```python
from build123d import *

# Parameters (mm, degrees)
ESBO_O1_R                = 175
RESSALTO_EXTRUS_O1_DEPTH = 97.5
ESBO_O4_R                = 1.5
ESBO_O4_R_2              = 2
CORTE_EXTRUS_O1_DEPTH    = 10
ESBO_O5_OUTSIDE_W        = 452.898
ESBO_O5_OUTSIDE_H        = 452.898
CORTE_EXTRUS_O2_DEPTH    = 8.4


with BuildPart() as part:
    # Esboço1 → Ressalto-extrusão1 (new body)
    with BuildSketch(Plane.XY):
        Circle(ESBO_O1_R)
    extrude(amount=RESSALTO_EXTRUS_O1_DEPTH)

    # Esboço4 → Corte-extrusão1 (cut)
    with BuildSketch(Plane.XY.offset(97.5)):
        with Locations((-120, 82)):
            Circle(ESBO_O4_R)
        with Locations((-55, 120)):
            Circle(ESBO_O4_R)
        with Locations((-77, 111.8)):
            Circle(ESBO_O4_R)
        with Locations((55, 120)):
            Circle(ESBO_O4_R)
        with Locations((-7, 111.8)):
            Circle(ESBO_O4_R_2)
        with Locations((-73, 80)):
            Circle(ESBO_O4_R_2)
        with Locations((21, 80)):
            Circle(ESBO_O4_R_2)
        with Locations(Location((21, -80, 0), (0, 0, 180))):
            Circle(ESBO_O4_R_2)
        with Locations(Location((-73, -80, 0), (0, 0, 180))):
            Circle(ESBO_O4_R_2)
        with Locations(Location((-7, -111.8, 0), (0, 0, 180))):
            Circle(ESBO_O4_R_2)
        with Locations(Location((55, -120, 0), (0, 0, 180))):
            Circle(ESBO_O4_R)
        with Locations(Location((-77, -111.8, 0), (0, 0, 180))):
            Circle(ESBO_O4_R)
        with Locations(Location((-55, -120, 0), (0, 0, 180))):
            Circle(ESBO_O4_R)
        with Locations(Location((-120, -82, 0), (0, 0, 180))):
            Circle(ESBO_O4_R)
    extrude(amount=-CORTE_EXTRUS_O1_DEPTH, mode=Mode.SUBTRACT)

    # Esboço5 outside → Corte-extrusão2 (cut)
    with BuildSketch(Plane.XY.offset(97.5)):
        Rectangle(ESBO_O5_OUTSIDE_W, ESBO_O5_OUTSIDE_H)
        with BuildLine():
            Line((28, -155.307222412), (120.5, -101.902322512))
            ThreePointArc((120.5, -101.902322512), (140.997422612, -81.4048999), (148.5, -53.4048999))
            Line((148.5, -53.4048999), (148.5, 53.4048999))
            ThreePointArc((148.5, 53.4048999), (140.997422612, 81.4048999), (120.5, 101.902322512))
            Line((120.5, 101.902322512), (28, 155.307222412))
            ThreePointArc((28, 155.307222412), (0, 162.8097998), (-28, 155.307222412))
            Line((-28, 155.307222412), (-120.5, 101.902322512))
            ThreePointArc((-120.5, 101.902322512), (-140.997422612, 81.4048999), (-148.5, 53.4048999))
            Line((-148.5, 53.4048999), (-148.5, -53.4048999))
            ThreePointArc((-148.5, -53.4048999), (-140.997422612, -81.4048999), (-120.5, -101.902322512))
            Line((-120.5, -101.902322512), (-28, -155.307222412))
            ThreePointArc((-28, -155.307222412), (0, -162.8097998), (28, -155.307222412))
        make_face(mode=Mode.SUBTRACT)
    extrude(amount=-CORTE_EXTRUS_O2_DEPTH, mode=Mode.SUBTRACT)


solid = part.part
```
Design review of the part built by this model. Coordinates are the model's own, in mm. A direction names the side the tool comes from. Give positions to 0.01 mm unless a question says otherwise; leave off trailing zeros. Write each loop counter-clockwise with the first axis right and the second up, starting at its lowest first coordinate (ties: lowest second). Pieces come first, ordered by that corner, then holes. Notation, with made-up numbers: (-1, 43.5) - (13, 43.5) arc R27 ccw to (13, 82.5) - close; hole circle Ø10 at (-17, -10). An arc over 180 degrees is marked (long way). Return JSON: item names as keys, results as strings. Group by question number.
(1) We need section C-C, the plane x = 139.5. Give the boundary of the cut face in (y, z).
(2) We need section B-B, the plane z = 39. Give the boundary of the cut face in (x, y), then the cut area to 3 significant figures.
(3) Machinability: for faces 1 (the flat face through (148.5, -1, 93)), 2 (the flat face through (73.6, -128.98, 93.36)), 3 (the flat face through (-79, -129, 89.1)), 4 (the cylindrical face through (-141.2, -81.05, 93.36)), which of the approach directions +Z, -Z, +X, -X, +Y, -Y give a long, thin tool a straight path to every point of the face, cutting with its end or side? Answer none if there is none.
(4) To check wall thickness, follow probe 1 along Y at (x, z) = (21, 93.25); probe 2 along X at (y, z) = (111, 90); probe 3 along Y at (x, z) = (-120, 93). State the ranges of each line that lie inside material, in increasing order.
(5) Insertion check: pin 1 (1.5 mm diameter, centred on x = 55.5, y = 120, fed in from +Z); pin 2 (4 mm diameter, centred on x = -9, z = 10, fed in from +Y); pin 3 (5 mm diameter, centred on x = -115.5, z = 49, fed in from -Y). Each pin has a flat end and moves straight along its axis. Give the tip position at first contact, or say it passes through.
(6) We need section A-A, the plane y = 39. Give the boundary of the cut face in (x, z).
Reported:
{
 "1": {"outline": "(-105.66, 0) - (105.66, 0) - (105.66, 89.1) - (83.85, 89.1) - (83.85, 97.5) - (-83.85, 97.5) - (-83.85, 89.1) - (-105.66, 89.1) - close"},
 "2": {"outline": "circle Ø350 at (0, 0)", "area": "96,200 mm2"},
 "3": {"face 1": "+Z, +X, +Y, -Y", "face 2": "+Z, +X, -Y", "face 3": "+Z", "face 4": "+Z, -X, -Y"},
 "4": {"probe 1": "y = -158.72 to -82, -78 to 78, 82 to 158.72", "probe 2": "x = -104.74 to -78.27, -75.73 to -8.83, -5.17 to 104.74", "probe 3": "y = -102.19 to -83.5, -80.5 to 80.5, 83.5 to 102.19"},
 "5": {"pin 1": "stops at z = 87.5", "pin 2": "stops at y = 174.86", "pin 3": "stops at y = -133.63"},
 "6": {"outline": "(-170.6, 0) - (170.6, 0) - (170.6, 89.1) - (148.5, 89.1) - (148.5, 97.5) - (-148.5, 97.5) - (-148.5, 89.1) - (-170.6, 89.1) - close"}
}
